Solid Edge part; units mm, degrees
sketch "Sketch1" plane through (0, 0, 0) normal (0, -1, 0) x (1, 0, 0)
  line L0 (-32.6578, 15.458) -> (32.6578, 15.458)
  line L1 (32.6578, 15.458) -> (32.6578, -15.458)
  line L2 (32.6578, -15.458) -> (-32.6578, -15.458)
  line L3 (-32.6578, -15.458) -> (-32.6578, 15.458)
extrude "Protrusion1" add sketch "Sketch1" against normal blind 85.0283
sketch "Sketch2" plane through (0, 42.5142, 15.458) normal (0, 0, 1) x (0, 1, 0)
  circle A0 centre (0, 0) radius 14.7818
extrude "Cutout1" cut sketch "Sketch2" against normal up to next
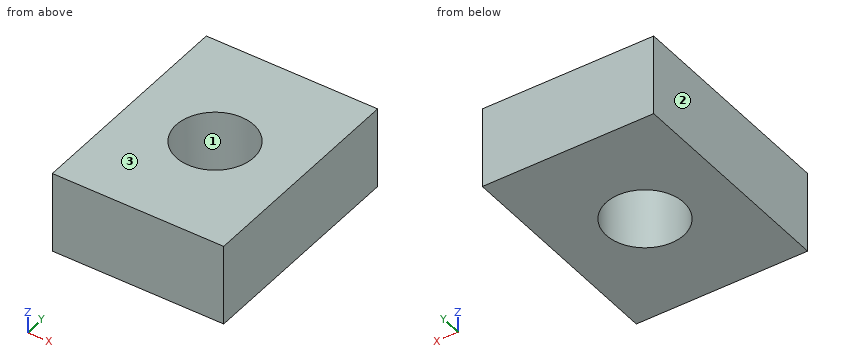
Model file for the job. Use its own axes, mm. Face numbers are marked on the shaded views. Give positions to 0.01 mm unless a question says otherwise; leave off trailing zeros. Loops run counter-clockwise (first coordinate to the right, second up) from the corner with the lowest first, then second, coordinate; pieces in that order, holes last.
1) Saw through at C-C (y = 36.5). Write the cut outline in (x, z).
2) Wall check: line 1 (Y direction, x = 0, z = 1); line 2 (X direction, y = 42.5, z = -2.5); line 3 (X direction, y = 39.5, z = 13). Give the ranges that are in metal, low to high.
3) Pull direction X, two halves, no side cores. Call the marked faces 1, 2 and 3: +X half, -X half, draft (parallel to the pull), parting line (faces both ways), or undercut.
4) Flat gauge pin, fed straight in: pin 1 Ø6 at (x, z) = (-11, 8.5) entering from -Y. Where does the tip first touch, or does it go through?
5) Saw through at A-A (x = 0). Write the cut outline in (y, z).
6) Saw through at B-B (z = 12). Write the cut outline in (x, y), plus the area to 3 significant figures.
Answer block:
1. outline: (-32.66, -15.46) - (-13.5, -15.46) - (-13.5, 15.46) - (-32.66, 15.46) - close; (13.5, -15.46) - (32.66, -15.46) - (32.66, 15.46) - (13.5, 15.46) - close
2. line 1: y = 0 to 27.73, 57.3 to 85.03
2. line 2: x = -32.66 to -14.78, 14.78 to 32.66
2. line 3: x = -32.66 to -14.47, 14.47 to 32.66
3. face 1: undercut
3. face 2: -X half
3. face 3: draft
4. pin 1: stops at y = 0
5. outline: (0, -15.46) - (27.73, -15.46) - (27.73, 15.46) - (0, 15.46) - close; (57.3, -15.46) - (85.03, -15.46) - (85.03, 15.46) - (57.3, 15.46) - close
6. outline: (-32.66, 0) - (32.66, 0) - (32.66, 85.03) - (-32.66, 85.03) - close; hole circle Ø29.56 at (0, 42.51)
6. area: 4,870 mm2
